The model under review builds one solid part; all positions refer to its coordinate system, in mm. A direction names the side the tool comes from. Coordinates: 2 decimals unless noted, no trailing zeros. Loops run counter-clockwise (first coordinate to the right, second up) from the corner with the lowest first, then second, coordinate; pieces in that order, holes last. Notation, with made-up numbers: (46.5, 51.25) - (52.5, 51.25) arc R27 cw to (52.5, 78.25) - close; hole circle Ø7 at (70.25, -12.75). An arc over 180 degrees is marked (long way). Use a Markdown table: item, result. Add a question column.
1) The part is to be moulded in two halves that separate along X. For faces 4 (the flat face through (-4.6, -9.8, 5.6)), 5 (the cylindrical face through (1.95, -9.76, 5.63)), 6 (the cylindrical face through (9.763, -1.932, 5.635)), say which applies: pulls with the +X half, pulls with the -X half, needs draft (parallel to the pull), parting line crosses it, or undercut.
2) Add section B-B, the plane x = -9.25. Give the boundary of the cut face in (y, z), and give its area (3 significant figures).
3) To check wall thickness, follow L1, parallel to Y at x = 0.25, z = 8.5; L2, parallel to Y at x = -0.25, z = 9.5; L3, parallel to Y at x = -5.5, z = 1. State the ranges of each line that lie inside material, in increasing order. Write a range as [from, to].
4) Add section A-A, the plane y = -0.5. Give the boundary of the cut face in (x, z).
5) For faces 1 (the flat face through (10.78, -0.52, 5.63)), 2 (the flat face through (-3.646, -10.182, 5.635)), 3 (the cylindrical face through (-9.763, 1.932, 5.635)), list the 3-axis set-ups (+Z, -Z, +X, -X, +Y, -Y) from which the entire face can be reached by the end or side of a thin tool; tool diameter is ignored.
6) Clearance check with flat-ended pins moving along their axes: pin 1 (1.5 mm diameter, centred on y = -3, z = 2, fed in from +X); pin 2 (6 mm diameter, centred on x = 5.5, z = 2, fed in from -Y); pin 3 (1.5 mm diameter, centred on y = 4, z = 3.5, fed in from -X). State where each tip first meets the part, or that it passes through.
```python
from build123d import *

# Parameters (mm, degrees)
F0_R     = 1.27
F1_DEPTH = 11.43


with BuildPart() as f1:
    # F0 (on Top) → F1 (new body)
    with BuildSketch(Plane.XY):
        with BuildLine():
            ThreePointArc((9.952559, 0), (9.93813, 0.535724), (9.894886, 1.069894))
            ThreePointArc((9.894886, 1.069894), (9.756852, 1.963995), (9.538198, 2.841867))
            ThreePointArc((9.538198, 2.841867), (9.18622, 3.829725), (8.732252, 4.775062))
            ThreePointArc((8.732252, 4.775062), (8.262568, 5.54828), (7.724611, 6.275654))
            ThreePointArc((7.724611, 6.275654), (7.021389, 7.053619), (6.240211, 7.75327))
            ThreePointArc((6.240211, 7.75327), (5.510382, 8.28789), (4.735021, 8.754028))
            ThreePointArc((4.735021, 8.754028), (3.787614, 9.203663), (2.798155, 9.551113))
            ThreePointArc((2.798155, 9.551113), (1.919291, 9.765744), (1.024567, 9.899682))
            ThreePointArc((1.024567, 9.899682), (-0.02279, 9.952533), (-1.069894, 9.894886))
            ThreePointArc((-1.069894, 9.894886), (-1.963995, 9.756852), (-2.841867, 9.538198))
            ThreePointArc((-2.841867, 9.538198), (-3.829725, 9.18622), (-4.775062, 8.732252))
            ThreePointArc((-4.775062, 8.732252), (-5.54828, 8.262568), (-6.275654, 7.724611))
            ThreePointArc((-6.275654, 7.724611), (-7.053619, 7.021389), (-7.75327, 6.240211))
            ThreePointArc((-7.75327, 6.240211), (-8.28789, 5.510382), (-8.754028, 4.735021))
            ThreePointArc((-8.754028, 4.735021), (-9.203663, 3.787614), (-9.551113, 2.798156))
            ThreePointArc((-9.551113, 2.798156), (-9.765744, 1.919291), (-9.899682, 1.024567))
            ThreePointArc((-9.899682, 1.024567), (-9.952533, -0.02279), (-9.894886, -1.069894))
            ThreePointArc((-9.894886, -1.069894), (-9.756852, -1.963995), (-9.538198, -2.841867))
            ThreePointArc((-9.538198, -2.841867), (-9.18622, -3.829725), (-8.732252, -4.775062))
            ThreePointArc((-8.732252, -4.775062), (-8.262568, -5.54828), (-7.724611, -6.275654))
            ThreePointArc((-7.724611, -6.275654), (-7.021389, -7.053619), (-6.240211, -7.75327))
            ThreePointArc((-6.240211, -7.75327), (-5.510382, -8.28789), (-4.735021, -8.754028))
            ThreePointArc((-4.735021, -8.754028), (-3.787614, -9.203663), (-2.798156, -9.551113))
            ThreePointArc((-2.798156, -9.551113), (-1.919291, -9.765744), (-1.024567, -9.899682))
            ThreePointArc((-1.024567, -9.899682), (0.02279, -9.952533), (1.069894, -9.894886))
            ThreePointArc((1.069894, -9.894886), (1.963995, -9.756852), (2.841867, -9.538198))
            ThreePointArc((2.841867, -9.538198), (3.829725, -9.18622), (4.775062, -8.732252))
            ThreePointArc((4.775062, -8.732252), (5.54828, -8.262568), (6.275654, -7.724611))
            ThreePointArc((6.275654, -7.724611), (7.053619, -7.021389), (7.75327, -6.240211))
            ThreePointArc((7.75327, -6.240211), (8.28789, -5.510382), (8.754028, -4.735021))
            ThreePointArc((8.754028, -4.735021), (9.203663, -3.787614), (9.551113, -2.798155))
            ThreePointArc((9.551113, -2.798155), (9.765744, -1.919291), (9.899682, -1.024567))
            ThreePointArc((9.899682, -1.024567), (9.939331, -0.512965), (9.952559, 0))
        make_face()
        Circle(F0_R, mode=Mode.SUBTRACT)
        with BuildLine():
            Line((-2.841867, 9.538198), (-4.471273, 10.794608))
            Line((-4.471273, 10.794608), (-4.775062, 8.732252))
            ThreePointArc((-4.775062, 8.732252), (-3.829725, 9.18622), (-2.841867, 9.538198))
        make_face()
        with BuildLine():
            Line((1.024567, 9.899682), (0, 11.684))
            Line((0, 11.684), (-1.069894, 9.894886))
            ThreePointArc((-1.069894, 9.894886), (-0.02279, 9.952533), (1.024567, 9.899682))
        make_face()
        with BuildLine():
            Line((4.735021, 8.754028), (4.471273, 10.794608))
            Line((4.471273, 10.794608), (2.798155, 9.551113))
            ThreePointArc((2.798155, 9.551113), (3.787614, 9.203663), (4.735021, 8.754028))
        make_face()
        with BuildLine():
            Line((7.724611, 6.275654), (8.261836, 8.261836))
            Line((8.261836, 8.261836), (6.240211, 7.75327))
            ThreePointArc((6.240211, 7.75327), (7.021389, 7.053619), (7.724611, 6.275654))
        make_face()
        with BuildLine():
            Line((9.538198, 2.841867), (10.794608, 4.471273))
            Line((10.794608, 4.471273), (8.732252, 4.775062))
            ThreePointArc((8.732252, 4.775062), (9.18622, 3.829725), (9.538198, 2.841867))
        make_face()
        with BuildLine():
            Line((9.899682, -1.024567), (11.684, 0))
            Line((11.684, 0), (9.894886, 1.069894))
            ThreePointArc((9.894886, 1.069894), (9.93813, 0.535724), (9.952559, 0))
            ThreePointArc((9.952559, 0), (9.939331, -0.512965), (9.899682, -1.024567))
        make_face()
        with BuildLine():
            Line((8.754028, -4.735021), (10.794608, -4.471273))
            Line((10.794608, -4.471273), (9.551113, -2.798155))
            ThreePointArc((9.551113, -2.798155), (9.203663, -3.787614), (8.754028, -4.735021))
        make_face()
        with BuildLine():
            Line((6.275654, -7.724611), (8.261836, -8.261836))
            Line((8.261836, -8.261836), (7.75327, -6.240211))
            ThreePointArc((7.75327, -6.240211), (7.053619, -7.021389), (6.275654, -7.724611))
        make_face()
        with BuildLine():
            Line((2.841867, -9.538198), (4.471273, -10.794608))
            Line((4.471273, -10.794608), (4.775062, -8.732252))
            ThreePointArc((4.775062, -8.732252), (3.829725, -9.18622), (2.841867, -9.538198))
        make_face()
        with BuildLine():
            Line((-1.024567, -9.899682), (0, -11.684))
            Line((0, -11.684), (1.069894, -9.894886))
            ThreePointArc((1.069894, -9.894886), (0.02279, -9.952533), (-1.024567, -9.899682))
        make_face()
        with BuildLine():
            Line((-4.735021, -8.754028), (-4.471273, -10.794608))
            Line((-4.471273, -10.794608), (-2.798156, -9.551113))
            ThreePointArc((-2.798156, -9.551113), (-3.787614, -9.203663), (-4.735021, -8.754028))
        make_face()
        with BuildLine():
            Line((-7.724611, -6.275654), (-8.261836, -8.261836))
            Line((-8.261836, -8.261836), (-6.240211, -7.75327))
            ThreePointArc((-6.240211, -7.75327), (-7.021389, -7.053619), (-7.724611, -6.275654))
        make_face()
        with BuildLine():
            Line((-9.538198, -2.841867), (-10.794608, -4.471273))
            Line((-10.794608, -4.471273), (-8.732252, -4.775062))
            ThreePointArc((-8.732252, -4.775062), (-9.18622, -3.829725), (-9.538198, -2.841867))
        make_face()
        with BuildLine():
            Line((-9.899682, 1.024567), (-11.684, 0))
            Line((-11.684, 0), (-9.894886, -1.069894))
            ThreePointArc((-9.894886, -1.069894), (-9.952533, -0.02279), (-9.899682, 1.024567))
        make_face()
        with BuildLine():
            Line((-8.754028, 4.735021), (-10.794608, 4.471273))
            Line((-10.794608, 4.471273), (-9.551113, 2.798156))
            ThreePointArc((-9.551113, 2.798156), (-9.203663, 3.787614), (-8.754028, 4.735021))
        make_face()
        with BuildLine():
            Line((-6.275654, 7.724611), (-8.261836, 8.261836))
            Line((-8.261836, 8.261836), (-7.75327, 6.240211))
            ThreePointArc((-7.75327, 6.240211), (-7.053619, 7.021389), (-6.275654, 7.724611))
        make_face()
    extrude(amount=F1_DEPTH)


solid = f1.part
```
From the geometry:
| question | item | result |
|---|---|---|
| 1 | face 4 | pulls with the -X half |
| 1 | face 5 | undercut |
| 1 | face 6 | pulls with the +X half |
| 2 | outline | (-4.7, 0) - (4.67, 0) - (4.67, 11.43) - (-4.7, 11.43) - close |
| 2 | area | 107 mm^2 |
| 3 | L1 | y = [-11.27, -1.25], [1.25, 11.25] |
| 3 | L2 | y = [-11.25, -1.25], [1.25, 11.27] |
| 3 | L3 | y = [-8.29, 8.29] |
| 4 | outline | (-10.85, 0) - (-1.17, 0) - (-1.17, 11.43) - (-10.85, 11.43) - close; (1.17, 0) - (10.81, 0) - (10.81, 11.43) - (1.17, 11.43) - close |
| 5 | face 1 | +Z, -Z, +X |
| 5 | face 2 | +Z, -Z, -Y |
| 5 | face 3 | +Z, -Z, -X |
| 6 | pin 1 | stops at x = 10.26 |
| 6 | pin 2 | stops at y = -10.79 |
| 6 | pin 3 | stops at x = -10.79 |
